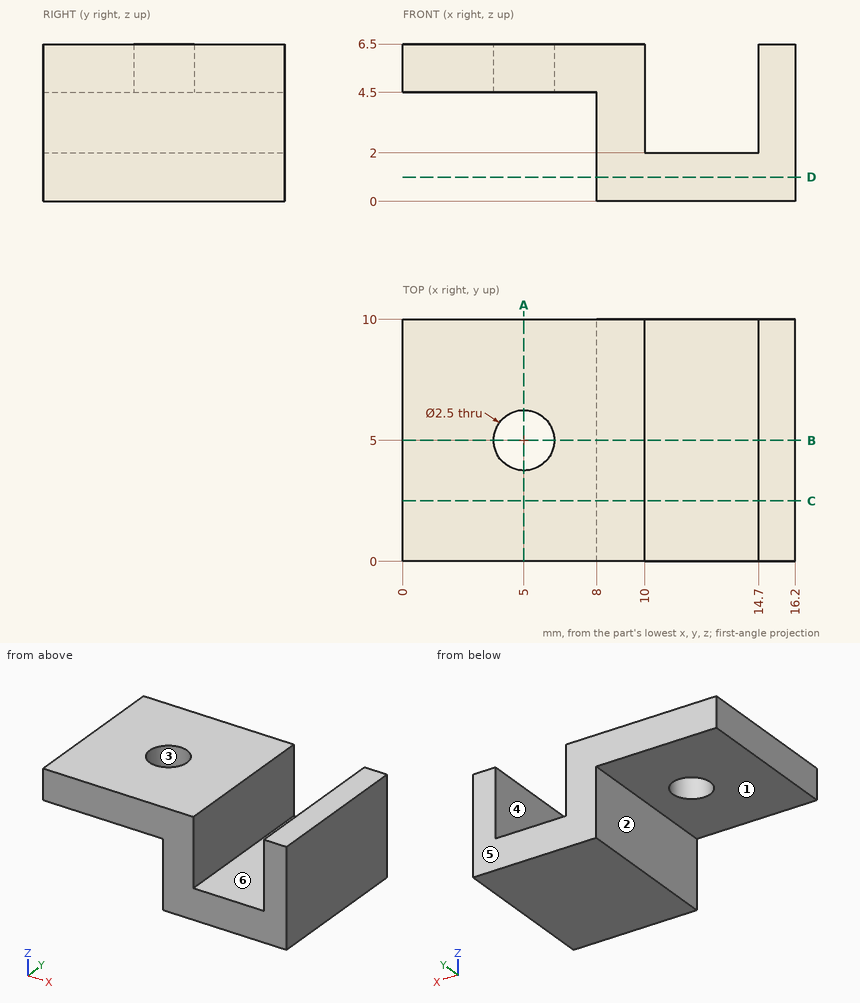
Input: dimensioned drawing with shaded views. Units: mm. Origin: part minimum x, y, z. A direction names the side the tool comes from. Coordinates: 2 decimals unless noted, no trailing zeros. Loops run counter-clockwise (first coordinate to the right, second up) from the corner with the lowest first, then second, coordinate; pieces in that order, holes last. Notation, with made-up numbers: M 69,48 L 82,48 A30 ccw 82,86 Z; hole C 81.5,-32.75 d3. An arc over 180 degrees is marked long. One line per item, written item: value.
(1) Section C-C (y = 2.5). Output: boundary loops of the cut face in (x, z), and give its area (4 significant figures).
Filled in:
outline: M 0,4.5 L 8,4.5 L 8,0 L 16.2,0 L 16.2,6.5 L 14.7,6.5 L 14.7,2 L 10,2 L 10,6.5 L 0,6.5 Z
area: 48.15 mm^2
(2) Reachability of the marked faces 5 and 6 from +Z, -Z, +X, -X, +Y, -Y: full face, straight path, thin tool, end or side. Return the list, or none.
Filled in:
face 5: +Z, -Z, +X, -X, +Y
face 6: +Z, +Y, -Y
(3) Pin query (flat end, axial travel): pin 1 (3.5 mm diameter, centred on y = 5.5, z = 2.5, fed in from -X). Return the tip coordinate at first contact, or that it passes through.
Filled in:
pin 1: x = 8
(4) Line query: line 1 along Y through (x, z) = (5, 6.05); line 2 along X through (y, z) = (4.5, 3.5); line 3 along Z through (x, y) = (5.5, 9.75). Output: solid intervals per line, ascending. Write a range as from..to.
Filled in:
line 1: 0..3.75, 6.25..10
line 2: 8..10, 14.7..16.2
line 3: 4.5..6.5
(5) Pull-direction query (X, two-part tool) for the marked faces 1, 2, 3 and 4; classes: +X half, -X half, draft (parallel to the pull), parting line (faces both ways), or undercut.
Filled in:
face 1: draft
face 2: -X half
face 3: undercut
face 4: undercut
(6) Section B-B (y = 5). Output: boundary loops of the cut face in (x, z).
Filled in:
outline: M 0,4.5 L 3.75,4.5 L 3.75,6.5 L 0,6.5 Z; M 6.25,4.5 L 8,4.5 L 8,0 L 16.2,0 L 16.2,6.5 L 14.7,6.5 L 14.7,2 L 10,2 L 10,6.5 L 6.25,6.5 Z
(7) Section D-D (z = 1). Output: boundary loops of the cut face in (x, y).
Filled in:
outline: M 8,0 L 16.2,0 L 16.2,10 L 8,10 Z
(8) Section A-A (x = 5). Output: boundary loops of the cut face in (y, z), and give its area (3 significant figures).
Filled in:
outline: M 0,4.5 L 3.75,4.5 L 3.75,6.5 L 0,6.5 Z; M 6.25,4.5 L 10,4.5 L 10,6.5 L 6.25,6.5 Z
area: 15.0 mm^2
